Work out the finished part from the listing and answer in its coordinate system (mm). Face numbers are marked on the shaded views. A direction names the side the tool comes from. Give positions to 0.01 mm unless a question says otherwise; leave off trailing zeros. Loops run counter-clockwise (first coordinate to the right, second up) from the corner with the lowest first, then second, coordinate; pieces in that order, holes last.
```python
from build123d import *

# Parameters (mm, degrees)
F0_W     = 175
F0_H     = 143
F1_DEPTH = 22
F2_T     = -2.5
F3_R     = 5


with BuildPart() as f1:
    # F0 (on Front) → F1 (new body)
    with BuildSketch(Plane.XZ):
        Rectangle(F0_W, F0_H)
    extrude(amount=F1_DEPTH)

    # F2
    f2_openings = [f1.faces().sort_by_distance(p)[0] for p in [
        (0, -22, 0),
    ]]
    offset(amount=F2_T, openings=f2_openings)

    # F3
    f3_edges = [f1.edges().sort_by_distance(p)[0] for p in [
        (-87.5, -11, 71.5),
        (-87.5, -11, -71.5),
        (87.5, -11, 71.5),
        (87.5, -11, -71.5),
    ]]
    fillet(f3_edges, radius=F3_R)


solid = f1.part
```
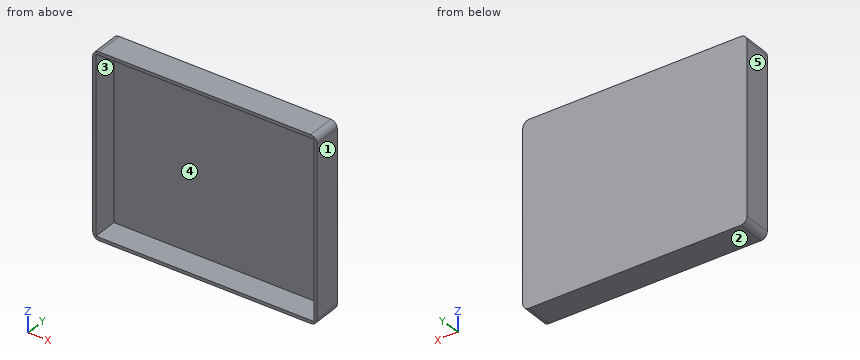
Q1. Determine the mould class of the marked faces 1, 2 and 3 for opening direction Z: +Z half, -Z half, draft (parallel to the pull), parting line (faces both ways), or undercut.
Q2. Section B-B on x = 0.5 is taken. Give the vertices of the cut face in (y, z), plus the area to 3 significant figures.
Q3. Section C-C on z = 45 is taken. Give the vertices of the cut face in (x, y).
Q4. Given pin 1 (1.5 mm diameter, centred on x = -42, z = -19, fed in from -Y), flat-ended and moving along its own axis, determine where the tip first touches the part or whether it passes through.
Q5. Consider line 1 along X through (y, z) = (-8.25, -0.5); line 2 along Z through (x, y) = (40.5, -6.75); line 3 along Y through (x, z) = (22, 10). Determine where each line is inside the solid, lowest interval first.
Q6. Which of the six approach directions +Z, -Z, +X, -X, +Y, -Y give full straight-line access (tool end or side, diameter ignored) to the marked faces 4 and 5?
Q7. Section A-A on y = -7.75 is taken. Give the vertices of the cut face in (x, z), plus the area to 3 significant figures.
Check result:
1. face 1: draft
1. face 2: -Z half
1. face 3: undercut
2. outline: (-22, -71.5) - (0, -71.5) - (0, 71.5) - (-22, 71.5) - (-22, 69) - (-2.5, 69) - (-2.5, -69) - (-22, -69) - close
2. area: 455 mm2
3. outline: (-87.5, -22) - (-85, -22) - (-85, -2.5) - (85, -2.5) - (85, -22) - (87.5, -22) - (87.5, 0) - (-87.5, 0) - close
4. pin 1: stops at y = -2.5
5. line 1: x = -87.5 to -85, 85 to 87.5
5. line 2: z = -71.5 to -69, 69 to 71.5
5. line 3: y = -2.5 to 0
6. face 4: -Y
6. face 5: +Z, -Z, -X, +Y, -Y
7. outline: (-87.5, -66.5) arc R5 ccw to (-82.5, -71.5) - (82.5, -71.5) arc R5 ccw to (87.5, -66.5) - (87.5, 66.5) arc R5 ccw to (82.5, 71.5) - (-82.5, 71.5) arc R5 ccw to (-87.5, 66.5) - close; hole (-85, -69) - (85, -69) - (85, 69) - (-85, 69) - close
7. area: 1,540 mm2
